Autodesk Fusion 360 part; units mm, degrees
sketch "Sketch1" plane through (0, 22, 0) normal (0, 1, 0) x (-1, 0, 0)
  line L0 (11.5698, 0.25) -> (15.3, 0.25)
  line L1 (15.3, 0.25) -> (15.3, -0.5)
  line L2 (15.3, -0.5) -> (15.6004, -0.5)
  line L3 (15.6004, -0.5) -> (15.6004, -1.2)
  line L4 (15.6004, -1.2) -> (16.0004, -1.2)
  line L5 (16.0004, -1.2) -> (16.0004, -0.5)
  line L6 (16.0004, -0.5) -> (16.3, -0.5)
  line L7 (16.3, -0.5) -> (16.3, 1.05)
  line L8 (16.3, 1.05) -> (5, 1.05)
  line L9 (11.5698, -1.2) -> (11.5698, 0.25)
  line L10 (11.5698, -0.6208) -> (11.2698, -0.6208) construction
  line L11 (11.2698, -0.5) -> (11.2698, -1.2)
  line L12 (11.2698, -0.5) -> (10.5698, -0.5)
  line L13 (10.5698, -0.5) -> (10.5698, -1.2)
  line L14 (10.5698, -0.678) -> (10.2698, -0.678) construction
  line L15 (10.2698, 1.05) -> (10.2698, -1.2)
  line L16 (10.2698, 1.05) -> (16.3, 1.05)
  line L17 (16.3, -0.5) -> (16.0004, -0.5)
  line L18 (16.0004, -1.2) -> (15.6004, -1.2)
  line L19 (15.6004, -0.5) -> (15.3, -0.5)
  line L20 (15.3, 0.25) -> (11.5698, 0.25)
  line L21 (11.5698, -1.2) -> (11.2698, -1.2)
  line L22 (11.5698, -1.2) -> (11.2698, -1.2)
  line L23 (11.2698, -0.5) -> (10.5698, -0.5)
  line L24 (10.5698, -1.2) -> (10.2698, -1.2)
  line L25 (10.2698, 1.05) -> (16.3, 1.05)
  line L26 (16.3, -0.5) -> (16.0004, -0.5)
  line L27 (16.0004, -1.2) -> (15.6004, -1.2)
  line L28 (15.6004, -0.5) -> (15.3, -0.5)
  line L29 (15.3, 0.25) -> (11.5698, 0.25)
  dimension "d14" = 0.3
  dimension "d15" = 0.7
  dimension "d16" = 0.3
extrude "Extrude1" add sketch "Sketch1" along normal blind 8.2 makes body 1
copy_body "Body->Comp1" bodies 1 removing the originals makes body 2 in component "Component"
move_face "OffsetFaces1" offset 0.3 1 faces at (-12.8132, 24.7333, 0.25) on bodies 2 in component "Component"
move_face "OffsetFaces2" offset -0.4 1 faces at (-12.2798, 27.4667, 1.05) on bodies 2 in component "Component"
move_face "OffsetFaces3" offset 3.3 1 faces at (-10.2698, 24.7333, 0.0333) on bodies 2 in component "Component"
move_face "OffsetFaces4" offset -3.3 1 faces at (-10.5698, 24.7333, -0.7333) on bodies 2 in component "Component"
move_face "OffsetFaces5" offset 3.3 1 faces at (-11.2698, 24.7333, -0.7333) on bodies 2 in component "Component"
move_face "OffsetFaces6" offset -3.3 1 faces at (-11.5698, 27.4667, -0.8167) on bodies 2 in component "Component"
move_face "OffsetFaces7" offset -4.2 1 faces at (-10.5132, 22, 0.4167) on bodies 2 in component "Component"
move_face "OffsetFaces8" offset -0.1 1 faces at (-8.2698, 28.8667, -0.4333) on bodies 2 in component "Component"
move_face "OffsetFaces9" offset 0.1 1 faces at (-7.9698, 27.5333, -0.7333) on bodies 2 in component "Component"
move_face "OffsetFaces10" offset 4.255 1 faces at (-10.4798, 26.2, 0.4167) on bodies 2 in component "Component"
move_face "OffsetFaces11" offset 0.3 1 faces at (-6.9698, 24.6967, 0.0333) on bodies 2 in component "Component"
move_face "OffsetFaces12" offset 0.3 1 faces at (-7.8698, 24.6967, -0.7333) on bodies 2 in component "Component"
move_face "OffsetFaces13" offset -0.3 1 faces at (-7.2698, 24.6967, -0.7333) on bodies 2 in component "Component"
move_face "OffsetFaces14" offset -0.3 1 faces at (-8.1698, 24.6967, -0.8167) on bodies 2 in component "Component"
move_face "OffsetFaces15" offset 1.8 2 faces at (-15.3, 24.6967, -0.2) (-15.6004, 24.6967, -0.7333) on bodies 2 in component "Component"
move_face "OffsetFaces16" offset -1.8 2 faces at (-16.0004, 24.6967, -0.9667) (-16.3, 24.6967, -0.1167) on bodies 2 in component "Component"
component "Component" placed x (1, 0, 0) y (0, 1, 0) z (0, 0, 1) at (0, 0, 0)
Design review of the part built by this model. Coordinates are the model's own, in mm. Round coordinates to 2 decimals unless told otherwise and drop trailing zeros. Order: outer loops, then holes, each group sorted by start corner. A loop starts at its lowest first (then second) coordinate and runs counter-clockwise, first axis right, second up. Notation, with made-up numbers: (-11.5, -20.5) - (37.5, -20.5) arc R26 cw to (37.5, 15.5) - close; hole circle Ø9 at (74, 50.5). An arc over 180 degrees is marked (long way). Return JSON: item names as keys, results as strings.
Q1. For pin 1 Ø0.7 at (x, y) = (-7, 26) entering from -Z; pin 2 Ø0.6 at (y, z) = (27, -1) entering from -X; pin 3 Ø1.7 at (x, y) = (-10.5, 28) entering from -Z, all flat-tipped, find the tip position at first contact; note any pin that passes through.
Computed values:
{"pin 1": "stops at z = -1.2", "pin 2": "stops at x = -14.2", "pin 3": "stops at z = -0.05"}
Q2. Wall thickness on L1, parallel to X at y = 27.5, z = -0.8; L2, parallel to Z at x = -10, y = 25.5; L3, parallel to X at y = 23.5, z = -0.3: over which ranges is each line inside the solid? List them lowest first. Write a range as [from, to].
Computed values:
{"L1": "x = [-14.2, -13.8], [-7.87, -7.57], [-6.97, -6.67]", "L2": "z = [-0.05, 0.65]", "L3": "x = [-14.5, -13.5], [-7.87, -6.67]"}
Q3. The part is to be moulded in two halves that separate along X. For faces 1 (the flat face through (-11, 26, -0.05)), 2 (the flat face through (-10.5, 21.945, 0.1)), 3 (the flat face through (-7.87, 26, -1)), 4 (the flat face through (-6.67, 26, 0)), say which applies: pulls with the +X half, pulls with the -X half, needs draft (parallel to the pull), parting line crosses it, or undercut.
Computed values:
{"face 1": "undercut", "face 2": "needs draft", "face 3": "undercut", "face 4": "pulls with the +X half"}
Q4. Consider section B-B on y = 29. Write out the cut boundary in (x, z), plus the area to 3 significant figures.
Computed values:
{"outline": "(-14.5, -0.5) - (-14.2, -0.5) - (-14.2, -1.2) - (-13.8, -1.2) - (-13.8, -0.5) - (-13.5, -0.5) - (-13.5, -0.05) - (-7.87, -0.05) - (-7.87, -1.2) - (-7.57, -1.2) - (-7.57, -0.5) - (-6.97, -0.5) - (-6.97, -1.2) - (-6.67, -1.2) - (-6.67, 0.65) - (-14.5, 0.65) - close", "area": "7.17 mm2"}
Q5. Consider section A-A on z = -0.4. Write out the cut boundary in (x, y) (3 decimals).
Computed values:
{"outline": "(-14.5, 21.945) - (-13.5, 21.945) - (-13.5, 30.2) - (-14.5, 30.2) - close; (-7.87, 21.945) - (-6.67, 21.945) - (-6.67, 30.2) - (-7.87, 30.2) - close"}
Q6. Consider section C-C on x = -13.25. Write out the cut boundary in (y, z) (3 decimals).
Computed values:
{"outline": "(21.945, -0.05) - (30.2, -0.05) - (30.2, 0.65) - (21.945, 0.65) - close"}
